Autodesk Fusion 360 part; units mm, degrees
sketch "Sketch1" plane through (0, 0, 0) normal (0, 0, 1) x (1, 0, 0)
  line L0 (-3.5, 17.5) -> (3.5, 17.5)
  line L1 (3.5, 17.5) -> (3.5, -17.5)
  line L2 (3.5, -17.5) -> (-3.5, -17.5)
  line L3 (-3.5, -17.5) -> (-3.5, 17.5)
  line L4 (-3.5, 17.5) -> (3.5, -17.5) construction
  line L5 (3.5, 17.5) -> (-3.5, -17.5) construction
  dimension "d13" = 7
  dimension "d14" = 35
extrude "Extrude1" add sketch "Sketch1" along normal blind 54.6
sketch "Sketch2" plane through (0, 0, 54.6) normal (0, 0, 1) x (-1, 0, 0)
  line L0 (3.5, 17.5) -> (-3.5, 17.5)
  line L1 (-3.5, 17.5) -> (-3.5, -17.5)
  line L2 (-3.5, -17.5) -> (3.5, -17.5)
  line L3 (3.5, -17.5) -> (3.5, 17.5)
  line L4 (-3.5, -17.5) -> (1.5, -17.5)
  line L5 (1.5, -17.5) -> (1.5, 12.5)
  line L6 (1.5, 12.5) -> (-3.5, 12.5)
  line L7 (-3.5, 12.5) -> (-3.5, -17.5)
  dimension "d17" = 5
  dimension "d18" = 30
extrude "Extrude2" cut sketch "Sketch2" against normal blind 54.6 contours L1 L2 L4 L5 L6 L7
sketch "Sketch3" plane through (0, 0, 54.6) normal (0, 0, 1) x (-1, 0, 0)
  line L0 (1.5, 12.5) -> (1.5, -17.5)
  line L1 (1.5, -17.5) -> (3.5, -17.5)
  line L2 (3.5, -17.5) -> (3.5, 17.5)
  line L3 (3.5, 17.5) -> (-3.5, 17.5)
  line L4 (-3.5, 17.5) -> (-3.5, 12.5)
  line L5 (-3.5, 12.5) -> (1.5, 12.5)
  line L6 (-1.5, 14.5) -> (3.5, 14.5)
  line L7 (3.5, 14.5) -> (3.5, 15.5)
  line L8 (3.5, 15.5) -> (-1.5, 15.5)
  line L9 (-1.5, 15.5) -> (-1.5, 14.5)
  dimension "d21" = 5
  dimension "d22" = 1
extrude "Extrude3" cut sketch "Sketch3" against normal blind 54.6 contours L2 L6 L7 L8 L9
Geometry check sheet. Reference: the model listing, model coordinates, mm. A direction names the side the tool comes from. Round coordinates to 2 decimals unless told otherwise and drop trailing zeros. Loops run counter-clockwise (first coordinate to the right, second up) from the corner with the lowest first, then second, coordinate; pieces in that order, holes last.
Item 1: Cross-section at A-A on x = -0.5. Record the boundary of the cut face in (y, z), then the cut area to 3 significant figures.
Item 2: Mould release check, pull along Y, two halves, no side actions. Record for faces 4 (the flat face through (-1, -15.5, 28)), 5 (the flat face through (-2, -3, 54.6)), 6 (the flat face through (0, -17.5, 27)): pulls with the +Y half, pulls with the -Y half, needs draft (parallel to the pull), parting line crosses it, or undercut.
Item 3: Cross-section at C-C on y = -2.5. Record the boundary of the cut face in (x, z).
Item 4: Access from +Z, -Z, +X, -X, +Y, -Y to the whole of each face (thin tool, end or side, straight path). Record for faces 1 (the flat face through (-2, -3, 0)), 2 (the flat face through (1.5, -15, 28)), 3 (the flat face through (1, -12.5, 28)).
Item 5: Gauge pin test, flat ends, axial feed: pin 1 (2.5 mm diameter, centred on x = 0, z = 20, fed in from +Y); pin 2 (3 mm diameter, centred on y = 0.5, z = 31, fed in from +X). Record the tip position at first contact, or that the pin passes through.
Item 6: Thickness scan on line 1 (Y direction, x = -2.5, z = 42); line 2 (Y direction, x = -1, z = 40); line 3 (Y direction, x = 2.75, z = 45). Record the ranges inside material, lowest first.
Item 7: Cross-section at D-D on x = 2.75. Record the boundary of the cut face in (y, z), then the cut area to 3 significant figures.
Item 8: Cross-section at B-B on z = 50. Record the boundary of the cut face in (x, y).
Answer sheet:
1. outline: (-17.5, 0) - (-15.5, 0) - (-15.5, 54.6) - (-17.5, 54.6) - close; (-14.5, 0) - (-12.5, 0) - (-12.5, 54.6) - (-14.5, 54.6) - close
1. area: 218 mm2
2. face 4: undercut
2. face 5: needs draft
2. face 6: pulls with the -Y half
3. outline: (-3.5, 0) - (-1.5, 0) - (-1.5, 54.6) - (-3.5, 54.6) - close
4. face 1: -Z, +X, -X, +Y, -Y
4. face 2: +Z, -Z, -X
4. face 3: +Z, -Z, +X, +Y
5. pin 1: stops at y = -12.5
5. pin 2: stops at x = -1.5
6. line 1: y = -17.5 to -15.5, -14.5 to 17.5
6. line 2: y = -17.5 to -15.5, -14.5 to -12.5
6. line 3: y = -17.5 to -12.5
7. outline: (-17.5, 0) - (-12.5, 0) - (-12.5, 54.6) - (-17.5, 54.6) - close
7. area: 273 mm2
8. outline: (-3.5, -17.5) - (3.5, -17.5) - (3.5, -12.5) - (-1.5, -12.5) - (-1.5, 17.5) - (-3.5, 17.5) - (-3.5, -14.5) - (1.5, -14.5) - (1.5, -15.5) - (-3.5, -15.5) - close
